Input: part model. Units: mm. Frame: model coordinates. Face numbers are marked on the shaded views. A direction names the side the tool comes from. Round coordinates to 2 decimals unless told otherwise and drop trailing zeros. Write each loop counter-clockwise with the first axis right and the second up, starting at its lowest first coordinate (ties: lowest second). Pieces come first, ordered by that corner, then holes. Notation, with made-up numbers: (10, 74) - (20, 74) arc R18 cw to (20, 105) - close; hole circle Ø6 at (27, -10). An arc over 180 degrees is marked (long way). One line per item, written item: value. Start each with the question number.
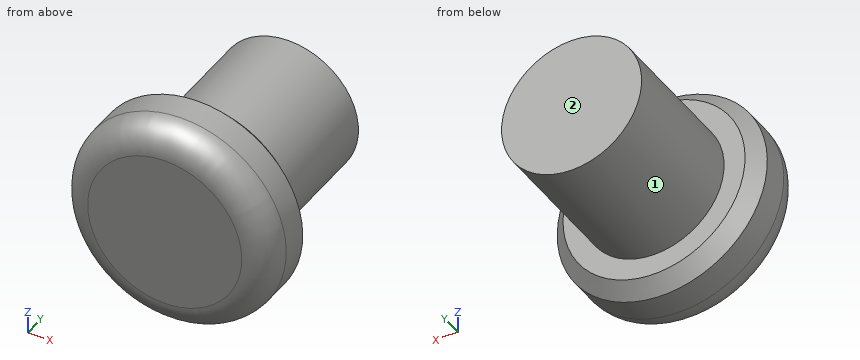
```python
from build123d import *

# Parameters (mm, degrees)
SKETCH1_R           = 7.5
BOSS_EXTRUDE1_DEPTH = 5
FILLET1_R           = 2
SKETCH2_R           = 5
BOSS_EXTRUDE2_DEPTH = 10
CHAMFER2_SIZE       = 1


with BuildPart() as part:
    # Sketch1 → Boss-Extrude1 (new body)
    with BuildSketch(Plane(origin=(0, 0, 0), x_dir=(1, 0, 0), z_dir=(0, 1, 0))):
        with Locations(Location((0, 0, 0), (0, 0, 270))):
            Circle(SKETCH1_R)
    extrude(amount=BOSS_EXTRUDE1_DEPTH)

    # Fillet1
    fillet1_edges = [part.edges().sort_by_distance(p)[0] for p in [
        (0, 0, -7.5),
    ]]
    fillet(fillet1_edges, radius=FILLET1_R)

    # Sketch2 → Boss-Extrude2 (add)
    with BuildSketch(Plane(origin=(0, 5, 0), x_dir=(1, 0, 0), z_dir=(0, 1, 0))):
        with Locations(Location((0, 0, 0), (0, 0, 270))):
            Circle(SKETCH2_R)
    extrude(amount=BOSS_EXTRUDE2_DEPTH)

    # Chamfer2
    chamfer2_edges = [part.edges().sort_by_distance(p)[0] for p in [
        (0, 5, -7.5),
    ]]
    chamfer(chamfer2_edges, length=CHAMFER2_SIZE)


solid = part.part
```
Q1. Access query for the marked faces 1 and 2. Directions: +Z, -Z, +X, -X, +Y, -Y. A direction counts if a zero-diameter tool reaches every point of the face in a straight line with its end or side. Return the directions, or none.
Q2. Cut plane C-C, the plane y = 1.5. Output: boundary loops of the cut face in (x, z), and give its area (3 significant figures).
Q3. Material intervals for probe 1 along Y at (x, z) = (-5, -1.25); probe 2 along Z at (x, y) = (1.75, 11.5); probe 3 along X at (y, z) = (1.75, -2.5), sorted ascending. Write a range as from..to.
Q4. Cut plane A-A, the plane z = 0. Output: boundary loops of the cut face in (x, y), and give its area (3 significant figures).
Q5. Contact query for flat-ended pins moving along their axis: pin 1 Ø5 at (y, z) = (2, -4.5) entering from +X; pin 2 Ø8 at (y, z) = (10, 5.5) entering from -X; pin 3 Ø1 at (y, z) = (4, -1) entering from -X. Output: stop coordinate, or through.
Q6. Cut plane B-B, the plane y = 7.25. Output: boundary loops of the cut face in (x, z), and give its area (3 significant figures).
A:
1. face 1: +Y
1. face 2: +Z, -Z, +X, -X, +Y
2. outline: circle Ø14.87 at (0, 0)
2. area: 174 mm²
3. probe 1: y = 0..5
3. probe 2: z = -4.68..4.68
3. probe 3: x = -7.05..7.05
4. outline: (-7.5, 2) arc R2 ccw to (-5.5, 0) - (5.5, 0) arc R2 ccw to (7.5, 2) - (7.5, 4) - (6.5, 5) - (5, 5) - (5, 15) - (-5, 15) - (-5, 5) - (-6.5, 5) - (-7.5, 4) - close
4. area: 172 mm²
5. pin 1: stops at x = 7.23
5. pin 2: stops at x = -4.77
5. pin 3: stops at x = -7.48
6. outline: circle Ø10 at (0, 0)
6. area: 78.5 mm²
